from build123d import *

# Parameters (mm, degrees)
BOSS_EXTRUDE2_DEPTH      = 12
BOSS_EXTRUDE2_DEPTH_BACK = 3
BOSS_EXTRUDE3_DEPTH      = 3
SKETCH8_W                = 4
SKETCH8_H                = 4
BOSS_EXTRUDE4_DEPTH      = 15
FILLET2_R                = 1.2
SKETCH9_R                = 0.75
CUT_EXTRUDE3_DEPTH       = 16
SKETCH10_R               = 3.5
CUT_EXTRUDE4_DEPTH       = 1.5
FILLET3_R                = 0.3
CUT_EXTRUDE5_DEPTH       = 12


with BuildPart() as part:
    # Sketch3 → Boss-Extrude2 (new body, two sides)
    with BuildSketch(Plane.XY) as boss_extrude2_sk:
        with BuildLine():
            Line((-69.81, 19.47), (-34.625063383, 19.47))
            ThreePointArc((-34.625063383, 19.47), (-32.763487521, 19.110531791), (-31.169582594, 18.083814123))
            Line((-31.169582594, 18.083814123), (-26.833005647, 13.937237175))
            ThreePointArc((-26.833005647, 13.937237175), (-26.514224661, 13.731893642), (-26.141909489, 13.66))
            Line((-26.141909489, 13.66), (-1.5, 13.66))
            ThreePointArc((-1.5, 13.66), (2.035533906, 12.195533906), (3.5, 8.66))
            Line((3.5, 8.66), (3.5, 1.5))
            ThreePointArc((3.5, 1.5), (2.035533906, -2.035533906), (-1.5, -3.5))
            Line((-1.5, -3.5), (-26.141909489, -3.5))
            ThreePointArc((-26.141909489, -3.5), (-26.514224661, -3.571893642), (-26.833005647, -3.777237175))
            Line((-26.833005647, -3.777237175), (-31.169582594, -7.923814123))
            ThreePointArc((-31.169582594, -7.923814123), (-32.763487521, -8.950531791), (-34.625063383, -9.31))
            Line((-34.625063383, -9.31), (-69.81, -9.31))
            ThreePointArc((-69.81, -9.31), (-73.345533906, -7.845533906), (-74.81, -4.31))
            Line((-74.81, -4.31), (-74.81, 14.47))
            ThreePointArc((-74.81, 14.47), (-73.345533906, 18.005533906), (-69.81, 19.47))
        make_face()
        with BuildLine():
            Line((-69.81, 17.47), (-34.625063383, 17.47))
            ThreePointArc((-34.625063383, 17.47), (-33.508117866, 17.254319075), (-32.55177491, 16.638288474))
            Line((-32.55177491, 16.638288474), (-28.215197962, 12.491711526))
            ThreePointArc((-28.215197962, 12.491711526), (-27.258855006, 11.875680925), (-26.141909489, 11.66))
            Line((-26.141909489, 11.66), (-1.5, 11.66))
            ThreePointArc((-1.5, 11.66), (0.621320344, 10.781320344), (1.5, 8.66))
            Line((1.5, 8.66), (1.5, 1.5))
            ThreePointArc((1.5, 1.5), (0.621320344, -0.621320344), (-1.5, -1.5))
            Line((-1.5, -1.5), (-26.141909489, -1.5))
            ThreePointArc((-26.141909489, -1.5), (-27.258855006, -1.715680925), (-28.215197962, -2.331711526))
            Line((-28.215197962, -2.331711526), (-32.55177491, -6.478288474))
            ThreePointArc((-32.55177491, -6.478288474), (-33.508117866, -7.094319075), (-34.625063383, -7.31))
            Line((-34.625063383, -7.31), (-69.81, -7.31))
            ThreePointArc((-69.81, -7.31), (-71.931320344, -6.431320344), (-72.81, -4.31))
            Line((-72.81, -4.31), (-72.81, 14.47))
            ThreePointArc((-72.81, 14.47), (-71.931320344, 16.591320344), (-69.81, 17.47))
        make_face(mode=Mode.SUBTRACT)
    extrude(amount=BOSS_EXTRUDE2_DEPTH)
    extrude(boss_extrude2_sk.sketch, amount=-BOSS_EXTRUDE2_DEPTH_BACK)

    # Sketch5 → Boss-Extrude3 (add)
    with BuildSketch(Plane(origin=(0, 0, -3), x_dir=(-1, 0, 0), z_dir=(0, 0, -1))):
        with BuildLine():
            Line((72.81, 14.47), (72.81, -4.31))
            ThreePointArc((72.81, -4.31), (71.931320344, -6.431320344), (69.81, -7.31))
            Line((69.81, -7.31), (34.625063383, -7.31))
            ThreePointArc((34.625063383, -7.31), (33.508117866, -7.094319075), (32.55177491, -6.478288474))
            Line((32.55177491, -6.478288474), (28.215197962, -2.331711526))
            ThreePointArc((28.215197962, -2.331711526), (27.258855006, -1.715680925), (26.141909489, -1.5))
            Line((26.141909489, -1.5), (1.5, -1.5))
            ThreePointArc((1.5, -1.5), (-0.621320344, -0.621320344), (-1.5, 1.5))
            Line((-1.5, 1.5), (-1.5, 8.66))
            ThreePointArc((-1.5, 8.66), (-0.621320344, 10.781320344), (1.5, 11.66))
            Line((1.5, 11.66), (26.141909489, 11.66))
            ThreePointArc((26.141909489, 11.66), (27.258855006, 11.875680925), (28.215197962, 12.491711526))
            Line((28.215197962, 12.491711526), (32.55177491, 16.638288474))
            ThreePointArc((32.55177491, 16.638288474), (33.508117866, 17.254319075), (34.625063383, 17.47))
            Line((34.625063383, 17.47), (69.81, 17.47))
            ThreePointArc((69.81, 17.47), (71.931320344, 16.591320344), (72.81, 14.47))
        make_face()
    extrude(amount=-BOSS_EXTRUDE3_DEPTH)

    # Sketch8 → Boss-Extrude4 (add, through all)
    with BuildSketch(Plane.XY.offset(12)):
        with Locations((-76.81, 12.47)):
            Rectangle(SKETCH8_W, SKETCH8_H)
        with Locations((-3.5, -5.5)):
            Rectangle(SKETCH8_W, SKETCH8_H)
    extrude(amount=-BOSS_EXTRUDE4_DEPTH)

    # Fillet2
    fillet2_edges = [part.edges().sort_by_distance(p)[0] for p in [
        (-74.81, 10.47, 4.5),
        (-78.81, 10.47, 4.5),
        (-78.81, 14.47, 4.5),
        (-1.5, -7.5, 4.5),
        (-5.5, -7.5, 4.5),
        (-5.5, -3.5, 4.5),
        (-1.5, -3.5, 4.5),
        (-74.81, 14.47, 4.5),
    ]]
    fillet(fillet2_edges, radius=FILLET2_R)

    # Sketch9 → Cut-Extrude3 (cut, through all)
    with BuildSketch(Plane.XY.offset(12)):
        with Locations((-76.81, 12.47)):
            Circle(SKETCH9_R)
        with Locations((-3.5, -5.5)):
            Circle(SKETCH9_R)
    extrude(amount=-CUT_EXTRUDE3_DEPTH, mode=Mode.SUBTRACT)

    # Sketch10 → Cut-Extrude4 (cut)
    with BuildSketch(Plane(origin=(0, 0, -3), x_dir=(-1, 0, 0), z_dir=(0, 0, -1))):
        with Locations((62.81, 5.08)):
            Circle(SKETCH10_R)
    extrude(amount=-CUT_EXTRUDE4_DEPTH, mode=Mode.SUBTRACT)

    # Fillet3
    fillet3_edges = [part.edges().sort_by_distance(p)[0] for p in [
        (-59.31, 5.08, -3),
    ]]
    fillet(fillet3_edges, radius=FILLET3_R)

    # Sketch11 → Cut-Extrude5 (cut)
    with BuildSketch(Plane.XY.offset(12)):
        with BuildLine():
            Line((-4.3, -7.5), (-2.7, -7.5))
            ThreePointArc((-2.7, -7.5), (-1.851471863, -7.148528137), (-1.5, -6.3))
            Line((-1.5, -6.3), (-1.5, -4.58276253))
            ThreePointArc((-1.5, -4.58276253), (-1.227013937, -3.820761768), (-0.532258065, -3.405453653))
            ThreePointArc((-0.532258065, -3.405453653), (2.362558069, -1.675003175), (3.5, 1.5))
            Line((3.5, 1.5), (3.5, 8.66))
            ThreePointArc((3.5, 8.66), (2.035533906, 12.195533906), (-1.5, 13.66))
            Line((-1.5, 13.66), (-26.141909489, 13.66))
            ThreePointArc((-26.141909489, 13.66), (-26.514224661, 13.731893642), (-26.833005647, 13.937237175))
            Line((-26.833005647, 13.937237175), (-31.169582594, 18.083814123))
            ThreePointArc((-31.169582594, 18.083814123), (-32.763487521, 19.110531791), (-34.625063383, 19.47))
            Line((-34.625063383, 19.47), (-69.81, 19.47))
            ThreePointArc((-69.81, 19.47), (-72.985003175, 18.332558069), (-74.715453653, 15.437741935))
            ThreePointArc((-74.715453653, 15.437741935), (-75.130761768, 14.742986063), (-75.89276253, 14.47))
            Line((-75.89276253, 14.47), (-77.61, 14.47))
            ThreePointArc((-77.61, 14.47), (-78.458528137, 14.118528137), (-78.81, 13.27))
            Line((-78.81, 13.27), (-78.81, 11.67))
            ThreePointArc((-78.81, 11.67), (-78.458528137, 10.821471863), (-77.61, 10.47))
            Line((-77.61, 10.47), (-76.01, 10.47))
            ThreePointArc((-76.01, 10.47), (-75.161471863, 10.118528137), (-74.81, 9.27))
            Line((-74.81, 9.27), (-74.81, -4.31))
            ThreePointArc((-74.81, -4.31), (-73.345533906, -7.845533906), (-69.81, -9.31))
            Line((-69.81, -9.31), (-34.625063383, -9.31))
            ThreePointArc((-34.625063383, -9.31), (-32.763487521, -8.950531791), (-31.169582594, -7.923814123))
            Line((-31.169582594, -7.923814123), (-26.833005647, -3.777237175))
            ThreePointArc((-26.833005647, -3.777237175), (-26.514224661, -3.571893642), (-26.141909489, -3.5))
            Line((-26.141909489, -3.5), (-6.7, -3.5))
            ThreePointArc((-6.7, -3.5), (-5.851471863, -3.851471863), (-5.5, -4.7))
            Line((-5.5, -4.7), (-5.5, -6.3))
            ThreePointArc((-5.5, -6.3), (-5.148528137, -7.148528137), (-4.3, -7.5))
        make_face()
        with BuildLine():
            Line((-69.81, -7.31), (-34.625063383, -7.31))
            ThreePointArc((-34.625063383, -7.31), (-33.508117866, -7.094319075), (-32.55177491, -6.478288474))
            Line((-32.55177491, -6.478288474), (-28.215197962, -2.331711526))
            ThreePointArc((-28.215197962, -2.331711526), (-27.258855006, -1.715680925), (-26.141909489, -1.5))
            Line((-26.141909489, -1.5), (-1.5, -1.5))
            ThreePointArc((-1.5, -1.5), (0.621320344, -0.621320344), (1.5, 1.5))
            Line((1.5, 1.5), (1.5, 8.66))
            ThreePointArc((1.5, 8.66), (0.621320344, 10.781320344), (-1.5, 11.66))
            Line((-1.5, 11.66), (-26.141909489, 11.66))
            ThreePointArc((-26.141909489, 11.66), (-27.258855006, 11.875680925), (-28.215197962, 12.491711526))
            Line((-28.215197962, 12.491711526), (-32.55177491, 16.638288474))
            ThreePointArc((-32.55177491, 16.638288474), (-33.508117866, 17.254319075), (-34.625063383, 17.47))
            Line((-34.625063383, 17.47), (-69.81, 17.47))
            ThreePointArc((-69.81, 17.47), (-71.931320344, 16.591320344), (-72.81, 14.47))
            Line((-72.81, 14.47), (-72.81, -4.31))
            ThreePointArc((-72.81, -4.31), (-71.931320344, -6.431320344), (-69.81, -7.31))
        make_face(mode=Mode.SUBTRACT)
    extrude(amount=-CUT_EXTRUDE5_DEPTH, mode=Mode.SUBTRACT)


solid = part.part
Source: CAD feature listing. Evaluate the final solid. Frame: model axes, mm. A direction names the side the tool comes from. Give positions to 0.01 mm unless a question says otherwise; leave off trailing zeros. Write each loop counter-clockwise with the first axis right and the second up, starting at its lowest first coordinate (ties: lowest second). Pieces come first, ordered by that corner, then holes. Notation, with made-up numbers: M -38.5,9 L -17.5,9 A27 cw -17.5,45 Z; hole C 70,30 d1. An arc over 180 degrees is marked long. Return JSON: item names as keys, results as strings. Group by question number.
1) Pull-direction query (X, two-part tool) for faces 1 (the face through (-4.095, -5.956, -1.479)), 2 (the face through (-28.97, -5.82, -1.48)), 3 (the face through (-4, -7.5, -1)), 4 (the face through (-1.5, -5, -1)); classes: pulls with the +X half, pulls with the -X half, needs draft (parallel to the pull), parting line crosses it, or undercut.
2) Cut plane D-D, the plane y = 5.08. Output: boundary loops of the cut face in (x, z).
3) Material intervals for line 1 along Y through (x, z) = (-76.81, -1.25); line 2 along Y through (x, z) = (-3.5, -1.55); line 3 along Y through (x, z) = (-12, -0.5), sorted ascending. Write a range as [from, to].
4) Cut plane A-A, the plane x = -3.5. Output: boundary loops of the cut face in (y, z).
5) Set-up query: faces 5 (the face through (-77, 14.47, -1)), 6 (the face through (-77, 10.47, -1)), 7 (the face through (-14, 13.66, -1)), 8 (the face through (-5.5, -6, -1)). Return all of +Z, -Z, +X, -X, +Y, -Y with unobstructed straight access to the full face (end or side cutting, diameter ignored); none if empty.
6) Cut plane C-C, the plane x = -62.81. Output: boundary loops of the cut face in (y, z).
7) Pin query (flat end, axial travel): P1, Ø2, axis at x = -61.5, y = 6, coming from the -Z side; P2, Ø0.5, axis at y = -5.5, z = -1.5, coming from the +X side; P3, Ø0.8, axis at x = -3.5, z = -1.5, coming from the -Y side. Return the tip coordinate at first contact, or that it passes through.
8) Cut plane B-B, the plane z = -2.15. Give the number of separate pieces and of enclosed holes in the cut face, plus the area to 3 significant figures.
Recorded:
{
 "1": {"face 1": "undercut", "face 2": "undercut", "face 3": "needs draft", "face 4": "pulls with the +X half"},
 "2": {"outline": "M -74.81,-3 L -66.61,-3 A0.3 ccw -66.31,-2.7 L -66.31,-1.5 L -59.31,-1.5 L -59.31,-2.7 A0.3 ccw -59.01,-3 L 3.5,-3 L 3.5,0 L -74.81,0 Z"},
 "3": {"line 1": "y = [10.47, 11.72], [13.22, 14.47]", "line 2": "y = [-7.5, -6.25], [-4.75, 13.66]", "line 3": "y = [-3.5, 13.66]"},
 "4": {"outline": "M -7.5,-3 L -6.25,-3 L -6.25,0 L -7.5,0 Z; M -4.75,-3 L 13.66,-3 L 13.66,0 L -4.75,0 Z"},
 "5": {"face 5": "+Z, -Z, -X, +Y", "face 6": "+Z, -Z, -X, -Y", "face 7": "+Z, -Z, +X, +Y", "face 8": "+Z, -Z, -Y"},
 "6": {"outline": "M -9.31,-3 L 1.28,-3 A0.3 ccw 1.58,-2.7 L 1.58,-1.5 L 8.58,-1.5 L 8.58,-2.7 A0.3 ccw 8.88,-3 L 19.47,-3 L 19.47,0 L -9.31,0 Z"},
 "7": {"P1": "stops at z = -1.5", "P2": "stops at x = -1.5", "P3": "stops at y = -7.5"},
 "8": {"separate pieces": "1", "enclosed holes": "3", "area": "1,840 mm²"}
}
